Verification items for the finished model (mm, model axes). A direction names the side the tool comes from. Round coordinates to 2 decimals unless told otherwise and drop trailing zeros. Loops run counter-clockwise (first coordinate to the right, second up) from the corner with the lowest first, then second, coordinate; pieces in that order, holes last. Notation, with made-up numbers: (31, 4) -> (65, 4) arc R7 ccw to (65, 14) -> close; hole circle Ø6 at (-10, 1.25). An arc over 180 degrees is marked (long way). Write item = value, one per line. Start each with the question number.
```python
from build123d import *

# Parameters (mm, degrees)
BOSS_EXTRU_1_DEPTH      = 25.5
ESQUISSE2_R             = 1.385
BOSS_EXTRU_2_DEPTH      = 4.7
ESQUISSE3_R             = 1.35
ENL_V_MAT_EXTRU_1_DEPTH = 4.7


with BuildPart() as part:
    # Esquisse1 → Boss.-Extru.1 (new body)
    with BuildSketch(Plane.XY):
        Polygon((3.550704156, 0), (1.775352078, 3.075), (-1.775352078, 3.075), (-3.550704156, 0), (-1.775352078, -3.075), (1.775352078, -3.075), align=None)
    extrude(amount=BOSS_EXTRU_1_DEPTH)

    # Esquisse2 → Boss.-Extru.2 (add)
    with BuildSketch(Plane.XY.offset(25.5)):
        Circle(ESQUISSE2_R)
    extrude(amount=BOSS_EXTRU_2_DEPTH)

    # Esquisse3 → Enlèv. mat.-Extru.1 (cut)
    with BuildSketch(Plane(origin=(0, 0, 0), x_dir=(-1, 0, 0), z_dir=(0, 0, -1))):
        Circle(ESQUISSE3_R)
    extrude(amount=-ENL_V_MAT_EXTRU_1_DEPTH, mode=Mode.SUBTRACT)


solid = part.part
```
(1) Section check B-B on z = 10.5. Enter the section's corners in (x, y) (3 decimals), then the cut area to 3 significant figures.
(2) Scan lines: line 1 (Y direction, x = 0, z = 2.85) (3 decimals); line 2 (Z direction, x = 1.75, y = -1); line 3 (Z direction, x = 0.5, y = -1). Record each from-to range of solid material in increasing order. Write a range as [from, to].
(3) Draft check along Y on faces 1 (the flat face through (0, 3.075, 13)), 2 (the flat face through (0, -3.075, 13)), 3 (the flat face through (0, 0, 4.7)). Enter one of: +Y half, -Y half, draft (parallel to the pull), parting line (faces both ways), or undercut.
(4) Section check A-A on x = 0. Enter the section's corners in (y, z) (3 decimals), then the cut area to 3 significant figures.
(5) Access from +Z, -Z, +X, -X, +Y, -Y to the whole of each face (thin tool, end or side, straight path). Record for faces 4 (the flat face through (0, 0, 30.2)), 5 (the cylindrical face through (0.29, -1.32, 2.32)), 6 (the cylindrical face through (1.32, 0.42, 27.82)).
(6) Section check C-C on y = 2. Enter the section's corners in (x, z), then the cut area to 3 significant figures.
(7) Depth check by flat-ended pin: pin 1 Ø1.5 at (x, y) = (2.5, -2) entering from +Z; pin 2 Ø2.5 at (x, y) = (0, 0) entering from -Z; pin 3 Ø1 at (x, z) = (-2, 12) entering from -Y (3 decimals). Enter the tip coordinate at first touch or a pass-through.
Computed values:
q1.outline = (-3.551, 0) -> (-1.775, -3.075) -> (1.775, -3.075) -> (3.551, 0) -> (1.775, 3.075) -> (-1.775, 3.075) -> close
q1.area = 32.8 mm²
q2.line_1 = [-3.075, -1.35], [1.35, 3.075]
q2.line_2 = [0, 25.5]
q2.line_3 = [4.7, 30.2]
q3.face_1 = +Y half
q3.face_2 = -Y half
q3.face_3 = undercut
q4.outline = (-3.075, 0) -> (-1.35, 0) -> (-1.35, 4.7) -> (1.35, 4.7) -> (1.35, 0) -> (3.075, 0) -> (3.075, 25.5) -> (1.385, 25.5) -> (1.385, 30.2) -> (-1.385, 30.2) -> (-1.385, 25.5) -> (-3.075, 25.5) -> close
q4.area = 157 mm²
q5.face_4 = +Z, +X, -X, +Y, -Y
q5.face_5 = -Z
q5.face_6 = +Z
q6.outline = (-2.4, 0) -> (2.4, 0) -> (2.4, 25.5) -> (-2.4, 25.5) -> close
q6.area = 122 mm²
q7.pin_1 = 25.5
q7.pin_2 = 4.7
q7.pin_3 = -3.075
